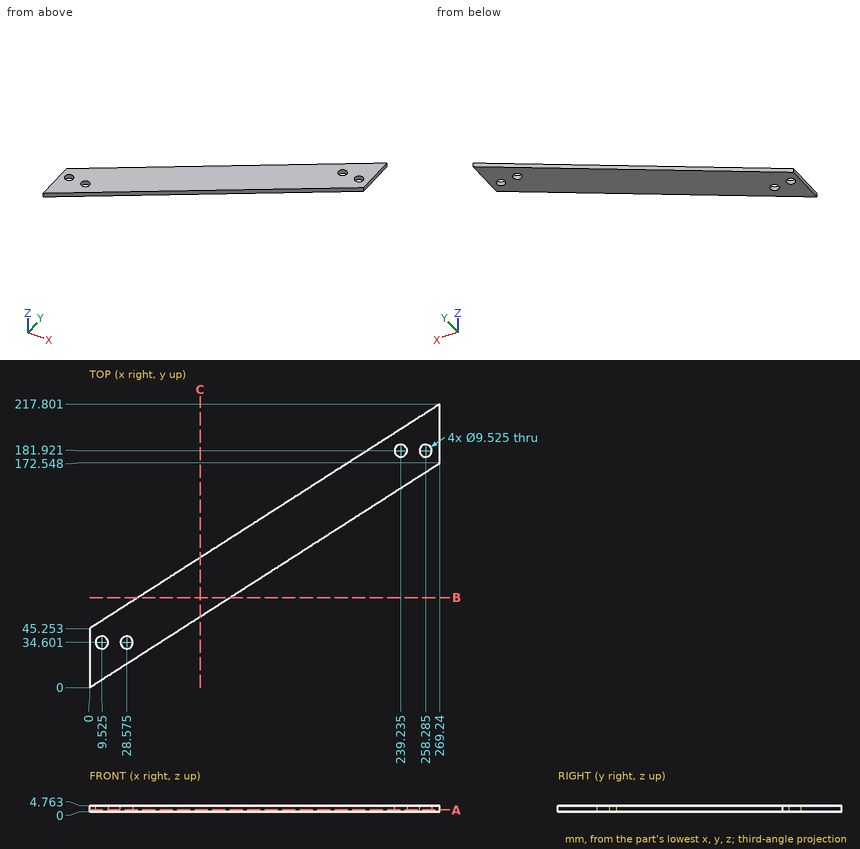
Here's the drawing with two shaded views (mm, measured from the low corner). I have some questions. Round coordinates to 2 decimals unless told otherwise and drop trailing zeros. Loops run counter-clockwise (first coordinate to the right, second up) from the corner with the lowest first, then second, coordinate; pieces in that order, holes last. Notation, with made-up numbers: M -4.75,73.5 L 34.25,73.5 A38 ccw 34.25,112.5 Z; hole C -37.5,14 d5. An arc over 180 degrees is marked long. Put each result on its own line as item: value.
Q1. Imagine slicing it at C-C (x = 85). Write out the boundary of the cut face in (y, z) (1 decimal).
Check result:
outline: M 54.5,0 L 99.7,0 L 99.7,4.8 L 54.5,4.8 Z
Q2. For pin 1 (1 mm diameter, centred on x = 151.5, z = 2.5, fed in from +Y) (1 decimal); pin 2 (1 mm diameter, centred on x = 193.5, z = 1, fed in from +Y), each with a flat end and sliding along its axis, tell me the tip position at first contact or that it passes through.
Check result:
pin 1: y = 142.7
pin 2: y = 169.58
Q3. Imagine slicing it at A-A (z = 1.5). Write out the boundary of the cut face in (x, y) (1 decimal).
Check result:
outline: M 0,0 L 269.2,172.5 L 269.2,217.8 L 0,45.3 Z; hole C 9.5,34.6 d9.5; hole C 28.6,34.6 d9.5; hole C 239.2,181.9 d9.5; hole C 258.3,181.9 d9.5
Q4. I need wall thicknesses on probe 1 along X at (y, z) = (179.5, 0.35) (1 decimal); probe 2 along X at (y, z) = (180.5, 4.2) (1 decimal); probe 3 along Y at (x, z) = (18, 1.35) (1 decimal). Which ranges of each line are inside material? Lowest first, please.
Check result:
probe 1: 209.5 to 235.1, 243.3 to 254.2, 262.4 to 269.2
probe 2: 211 to 234.7, 243.8 to 253.7, 262.8 to 269.2
probe 3: 11.5 to 56.8
Q5. Imagine slicing it at B-B (y = 69). Write out the boundary of the cut face in (x, z) (1 decimal).
Check result:
outline: M 37.1,0 L 107.7,0 L 107.7,4.8 L 37.1,4.8 Z
